Autodesk Inventor part; units mm, degrees
ref_plane "YZ Plane" through (0, 0, 0) normal (1, 0, 0) x (0, 1, 0)
ref_plane "XZ Plane" through (0, 0, 0) normal (0, 1, 0) x (-1, 0, 0)
ref_plane "XY Plane" through (0, 0, 0) normal (0, 0, 1) x (1, 0, 0)
sketch "Sketch1" plane through (0, 0, 0) normal (0, 1, 0) x (-1, 0, 0)
  line L0 (12.5, 25.5) -> (-12.5, 25.5)
  line L1 (-12.5, 25.5) -> (-12.5, -25.5)
  line L2 (-12.5, -25.5) -> (12.5, -25.5)
  line L3 (12.5, -25.5) -> (12.5, 25.5)
  line L4 (13, 26) -> (-13, 26)
  line L5 (-13, 26) -> (-13, -26)
  line L6 (-13, -26) -> (13, -26)
  line L7 (13, -26) -> (13, 26)
  line L8 (15, 28) -> (-15, 28)
  line L9 (-15, 28) -> (-15, -28)
  line L10 (-15, -28) -> (15, -28)
  circle A0 centre (8.5, 21.5) radius 2
  circle A1 centre (8.5, -21.5) radius 2
  circle A2 centre (-8.5, 21.5) radius 2
  circle A3 centre (-8.5, -21.5) radius 2
  line L11 (15, -28) -> (38, -28)
  line L12 (38, -28) -> (38, -26)
  line L13 (38, -26) -> (13, -26)
  line L14 (13, 26) -> (38, 26)
  line L15 (38, 26) -> (38, 28)
  line L16 (38, 28) -> (15, 28)
  line L17 (38, -26) -> (38, 26)
  line L18 (12.5, -15.5) -> (-12.5, -15.5)
  line L19 (12.5, 15.5) -> (-12.5, 15.5)
  line L20 (12.5, -15.5) -> (13, -15.5)
  line L21 (12.5, 15.5) -> (13, 15.5)
  line L22 (-12.5, -15.5) -> (-13, -15.5)
  line L23 (-12.5, 15.5) -> (-13, 15.5)
  point P0 (0, 0)
  dimension "d0" = 51
  dimension "d1" = 25
  dimension "d2" = 12.5
  dimension "d3" = 25.5
  dimension "d4" = 4
  dimension "d5" = 4
  dimension "d6" = 4
  dimension "d7" = 4
  dimension "d8" = 0.5
  dimension "d10" = 4
  dimension "d11" = 4
  dimension "d12" = 4
  dimension "d13" = 4
  dimension "d50" = 25
  dimension "d51" = 10
  dimension "d52" = 10
extrude "Extrusion1" add sketch "Sketch1" against normal blind 10 contours L3 L19 L1 L0 | L0 L1 L23 L5 L4 L7 L21 L3 | L21 L7 L20 L3 | L3 L18 L1 L19 | L1 L22 L5 L23 | L20 L7 L6 L5 L22 L1 L2 L3 | L3 L2 L1 L18 | L7 L14 L17 L13 | L5 L6 L13 L12 L11 L10 L9 L8 L16 L15 L14 L4 | A0 | A1 | A2 | A3
extrude "Extrusion2" add sketch "Sketch1" along normal blind 7 contours L5 L6 L13 L12 L11 L10 L9 L8 L16 L15 L14 L4
extrude "Extrusion3" cut sketch "Sketch1" against normal blind 6 contours A0 | A1 | A2 | A3
extrude "Extrusion8" cut sketch "Sketch1" against normal blind 7 contours L21 L7 L20 L3 | L3 L18 L1 L19 | L1 L22 L5 L23 | L7 L14 L17 L13
fillet "Fillet3" radius 2 6 edges at (-13, -3.5, -15.5) (-13, -3.5, -26) (13, -3.5, -15.5) (13, -3.5, 15.5) (-13, -3.5, 15.5) (-13, -3.5, 26)
sketch "Sketch7" plane through (8.5, -6, -21.5) normal (0, 1, 0) x (1, 0, 0)
  circle A0 centre (0, 0) radius 2
  circle A1 centre (-17, 0) radius 2
  circle A2 centre (-17, -43) radius 2
  circle A3 centre (0, -43) radius 2
  point P0 (-8.5, -21.5)
extrude "Extrusion9" cut sketch "Sketch7" against normal blind 1
sketch "Sketch8" plane through (-38, -10, -28) normal (-1, 0, 0) x (0, 0, 1)
  line L0 (54, 17) -> (54, 3)
  line L1 (54, 3) -> (2, 3)
  line L2 (2, 3) -> (2, 17)
  line L3 (0, 17) -> (2, 17)
  line L4 (0, 17) -> (0, 0)
  line L5 (56, 0) -> (0, 0)
  line L6 (56, 0) -> (56, 17)
  line L7 (54, 17) -> (56, 17)
  line L8 (2, 17) -> (54, 17)
  line L9 (13.7, 17) -> (13.7, 9)
  line L10 (13.7, 9) -> (19.7, 9)
  line L11 (19.7, 9) -> (19.7, 17)
  line L12 (36.7, 17) -> (36.7, 9)
  line L13 (36.7, 9) -> (42.7, 9)
  line L14 (42.7, 9) -> (42.7, 17)
  point P0 (28, 10)
  dimension "d58" = 6
  dimension "d59" = 6
  dimension "d60" = 17
  dimension "d63" = 11.7
  dimension "d66" = 8
extrude "Extrusion10" add sketch "Sketch8" against normal blind 2 contours L0 L1 L2 L8 L9 L10 L11 L12 L13 L14
fillet "Fillet4" radius 2 8 edges at (-37, -1, -14.3) (-37, -1, -8.3) (-37, -1, 8.7) (-37, -1, 14.7) (-38, -1.5, 28) (15, -1.5, 28) (15, -1.5, -28) (-38, -1.5, -28)
fillet "Fillet5" radius 2 2 edges at (-36, 0, -26) (-36, 0, 26)
sketch "Sketch10" plane through (0, -10, 0) normal (0, -1, 0) x (1, 0, 0)
  line L0 (-15, 26) -> (-34, 26)
  arc A0 (-34, 26) -> (-36, 24) centre (-34, 24) ccw
  line L1 (-36, -24) -> (-36, 24)
  arc A1 (-36, -24) -> (-34, -26) centre (-34, -24) ccw
  line L2 (-34, -26) -> (-15, -26)
  arc A2 (-38, -26) -> (-36, -28) centre (-36, -26) ccw
  line L3 (-36, -28) -> (13, -28)
  arc A3 (13, -28) -> (15, -26) centre (13, -26) ccw
  line L4 (15, -26) -> (15, 26)
  arc A4 (15, 26) -> (13, 28) centre (13, 26) ccw
  line L5 (13, 28) -> (-36, 28)
  arc A5 (-36, 28) -> (-38, 26) centre (-36, 26) ccw
  line L6 (-38, 26) -> (-38, -26)
  line L7 (-36, 24) -> (-36, 28)
  line L8 (-36, -24) -> (-36, -28)
  line L9 (-15, 28) -> (-15, -28)
  point P0 (0, 0)
extrude "Extrusion11" add sketch "Sketch10" along normal blind 20 contours L9 L2 A1 L1 A0 L0 | L0 A0 L7 L5 L9 | L9 L3 L8 A1 L2 | L1 L8 A2 L6 A5 L7
sketch "Sketch11" plane through (-38, 7, -8.3) normal (-1, 0, 0) x (0, 0, 1)
  line L0 (-17.7, -37) -> (-17.7, 0)
  line L1 (34.3, -37) -> (-17.7, -37)
  line L2 (34.3, 0) -> (34.3, -37)
  line L3 (34.3, 0) -> (23, 0)
  line L4 (23, 0) -> (23, -6)
  arc A0 (21, -8) -> (23, -6) centre (21, -6) ccw
  line L5 (21, -8) -> (19, -8)
  arc A1 (17, -6) -> (19, -8) centre (19, -6) ccw
  line L6 (17, -6) -> (17, 0)
  line L7 (17, 0) -> (0, 0)
  line L8 (0, 0) -> (0, -6)
  arc A2 (-2, -8) -> (0, -6) centre (-2, -6) ccw
  line L9 (-2, -8) -> (-4, -8)
  arc A3 (-6, -6) -> (-4, -8) centre (-4, -6) ccw
  line L10 (-6, -6) -> (-6, 0)
  line L11 (-17.7, 0) -> (-6, 0)
  arc A4 (23.2917, -37) -> (-6.6917, -37) centre (8.3, -37.5) ccw
  point P0 (8.3, -7)
  dimension "d71" = 52
  dimension "d72" = 26
  dimension "d73" = 0.5
  dimension "d74" = 30
extrude "Extrusion12" cut sketch "Sketch11" against normal through all contours A4 L1
fillet "Fillet6" radius 2 2 edges at (-15, -20, 28) (-15, -20, -28)
sketch "Sketch12" plane through (0, -30, 0) normal (0, -1, 0) x (1, 0, 0)
  arc A0 (-15, 26) -> (-17, 28) centre (-17, 26) ccw
  line L0 (-17, 28) -> (-36, 28)
  arc A1 (-36, 28) -> (-38, 26) centre (-36, 26) ccw
  line L1 (-38, 26) -> (-38, 14.9917)
  line L2 (-38, 14.9917) -> (-15, 14.9917)
  line L3 (-15, 14.9917) -> (-15, 26)
  arc A2 (-17, -28) -> (-15, -26) centre (-17, -26) ccw
  line L4 (-15, -26) -> (-15, -14.9917)
  line L5 (-15, -14.9917) -> (-38, -14.9917)
  line L6 (-38, -14.9917) -> (-38, -26)
  arc A3 (-38, -26) -> (-36, -28) centre (-36, -26) ccw
  line L7 (-36, -28) -> (-17, -28)
  point P0 (0, 0)
  point P1 (-26.5, 21.5)
  point P2 (-26.5, -21.5)
  dimension "d78" = 23
  dimension "d79" = 11.5
  dimension "d80" = 13.0083
  dimension "d81" = 6.5
  dimension "d82" = 6.5
hole "Hole1" at (-26.5, -30, 21.5) at (-26.5, -30, -21.5) direction (0, 1, 0) diameter 4.2 end through all
sketch "Sketch13" plane through (0, 7, 0) normal (0, 1, 0) x (1, 0, 0)
  line L0 (-47.6538, 31.9961) -> (20.3258, 31.9961)
  line L1 (20.3258, 31.9961) -> (20.3258, -36.2753)
  line L2 (20.3258, -36.2753) -> (-47.6538, -36.2753)
  line L3 (-47.6538, -36.2753) -> (-47.6538, 31.9961)
  point P0 (0, 0)
extrude "Extrusion13" cut sketch "Sketch13" against normal up to surface (17 mm away)
equation "\"d59\" = d58"
properties part number "3DP_ASA_Preamp_Case_Clamp"
For this review, take the finished solid that the model builds, in its own axes (mm). Round coordinates to 2 decimals unless told otherwise and drop trailing zeros. Order: outer loops, then holes, each group sorted by start corner. A loop starts at its lowest first (then second) coordinate and runs counter-clockwise, first axis right, second up. Notation, with made-up numbers: M -35,-28 L -28,-28 A13 ccw -28,-23 Z; hole C -9.5,87 d9. An arc over 180 degrees is marked long. Use a Markdown table: item, result. Add a question column.
Item 1: Mouldability with a two-part tool opening along Z and no side actions: class faces 1 (the cylindrical face through (-37.43, -19.86, 27.4)), 2 (the flat face through (-27, -10, 0)), 3 (the cylindrical face through (-26.661, -15.503, 0.323)) as released by +Z, released by -Z, zero draft, split by the parting line, or undercut.
Item 2: Add section C-C, the plane z = -21.5. Give the boundary of the cut face in (x, y).
Item 3: Add section B-B, the plane y = -12. Give the boundary of the cut face in (x, z).
Item 4: Add section A-A, the plane x = -26.5. Give the boundary of the cut face in (y, z), then the cut area to 3 significant figures.
Item 5: To check wall thickness, follow line 1 along Z through (x, y) = (-26.5, -14.25); line 2 along X through (y, z) = (-19.5, 21.5); line 3 along Z through (x, y) = (-27, -21.75). State the ranges of each line that lie inside material, in increasing order.
Item 6: Insertion check: pin 1 (5.5 mm diameter, centred on x = -26.5, z = -21.5, fed in from +Y). The pin has a flat end and moves straight along its axis. Give the tip position at first contact, or say it passes through.
Item 7: Add section D-D, the plane y = -25.5. Give the boundary of the cut face in (x, z).
Geometry results:
| question | item | result |
|---|---|---|
| 1 | face 1 | released by +Z |
| 1 | face 2 | zero draft |
| 1 | face 3 | undercut |
| 2 | outline | M -38,-30 L -28.6,-30 L -28.6,-10 L -38,-10 Z; M -24.4,-30 L -15,-30 L -15,-10 L -24.4,-10 Z |
| 3 | outline | M -38,-26 A2 ccw -36,-28 L -17,-28 A2 ccw -15,-26 L -15,26 A2 ccw -17,28 L -36,28 A2 ccw -38,26 Z; hole C -26.5,-21.5 d4.2; hole C -26.5,21.5 d4.2 |
| 4 | outline | M -30,-28 L -10,-28 L -10,-23.6 L -30,-23.6 Z; M -30,-19.4 L -10,-19.4 L -10,19.4 L -30,19.4 L -30,14.99 A15 cw -30,-14.99 Z; M -30,23.6 L -10,23.6 L -10,28 L -30,28 Z |
| 4 | area | 614 mm² |
| 5 | line 1 | z = -28 to -23.6, -19.4 to 19.4, 23.6 to 28 |
| 5 | line 2 | x = -38 to -28.6, -24.4 to -15 |
| 5 | line 3 | z = -28 to -23.54, -19.46 to -12.18, 12.18 to 19.46, 23.54 to 28 |
| 6 | pin 1 | stops at y = -10 |
| 7 | outline | M -38,-26 A2 ccw -36,-28 L -17,-28 A2 ccw -15,-26 L -15,-14.14 L -38,-14.14 Z; M -38,14.14 L -15,14.14 L -15,26 A2 ccw -17,28 L -36,28 A2 ccw -38,26 Z; hole C -26.5,-21.5 d4.2; hole C -26.5,21.5 d4.2 |
